Here's the drawing with two shaded views (mm, measured from the low corner). I have some questions. Coordinates: 2 decimals unless noted, no trailing zeros. Write each loop counter-clockwise with the first axis right and the second up, starting at its lowest first coordinate (ties: lowest second). Pieces come first, ordered by that corner, then holes. Notation, with made-up numbers: M -16,71.5 L 17,71.5 A31 cw 17,107.5 Z; hole C 13,-2.75 d10. An arc over 180 degrees is marked long. Answer as CSV lines item,"result". Start each with the question number.
Item 1: Suppose I cut it at B-B, the plane z = 0.4. State how many separate pieces and enclosed holes the cut face has, and give its area (3 significant figures).
Item 2: If I drill on line 1 along X through (y, z) = (82.4, 0.5); line 2 along X through (y, z) = (5, 0.9); line 3 along Y through (x, z) = (29.5, 0.45), over which ranges is the centre line in solid material (lowest first)? Write a range as [from, to].
Item 3: I'm going to push flat-ended pins straight in: P1, Ø0.8, axis at x = 40, z = 0.5, coming from the +Y side; P2, Ø0.8, axis at y = 66, z = 1, coming from the +X side; P3, Ø0.8, axis at y = 62.5, z = 1, coming from the -X side. Where does each tip first touch, or does it pass through?
Item 4: Suppose I cut it at C-C, the plane x = 12. Write out the boundary of the cut face in (y, z).
Item 5: Suppose I cut it at A-A, the plane y = 5. Write out the boundary of the cut face in (x, z).
Item 6: Suppose I cut it at D-D, the plane y = 48.5. Write out the boundary of the cut face in (x, z).
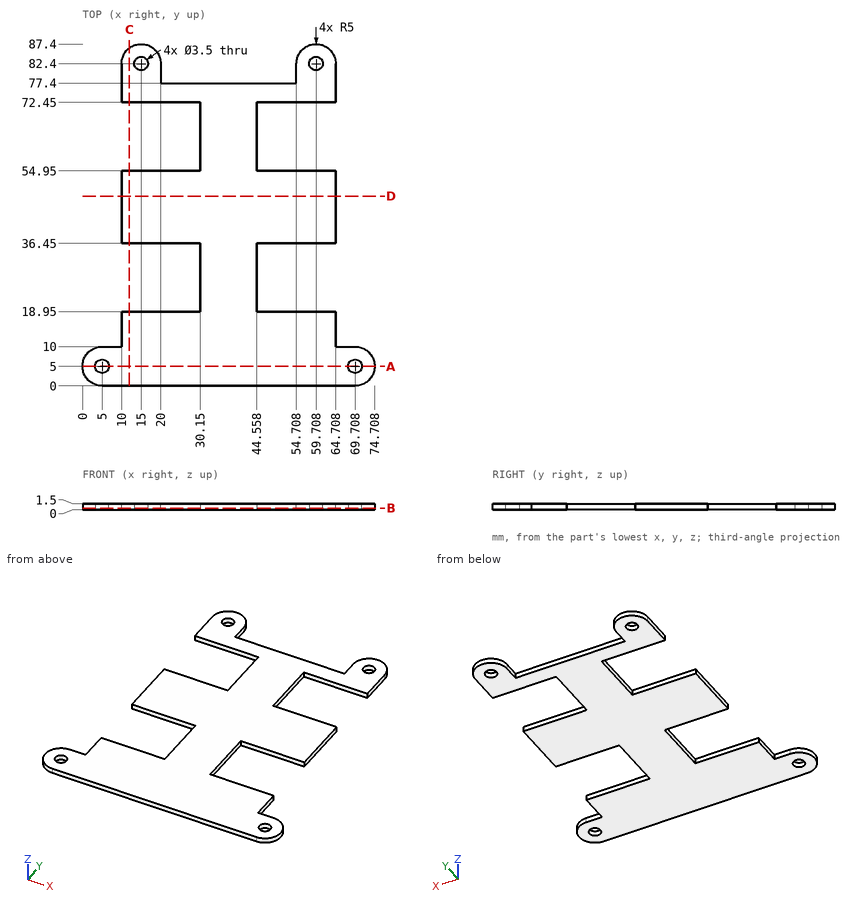
Ans:
1,separate pieces,"1"
1,enclosed holes,"4"
1,area,"3,140 mm^2"
2,line 1,"x = [10, 13.25], [16.75, 20], [54.71, 57.96], [61.46, 64.71]"
2,line 2,"x = [0, 3.25], [6.75, 67.96], [71.46, 74.71]"
2,line 3,"y = [0, 18.95], [36.45, 54.95], [72.45, 77.4]"
3,P1,"stops at y = 77.4"
3,P2,"stops at x = 44.56"
3,P3,"stops at x = 30.15"
4,outline,"M 0,0 L 18.95,0 L 18.95,1.5 L 0,1.5 Z; M 36.45,0 L 54.95,0 L 54.95,1.5 L 36.45,1.5 Z; M 72.45,0 L 86.4,0 L 86.4,1.5 L 72.45,1.5 Z"
5,outline,"M 0,0 L 3.25,0 L 3.25,1.5 L 0,1.5 Z; M 6.75,0 L 67.96,0 L 67.96,1.5 L 6.75,1.5 Z; M 71.46,0 L 74.71,0 L 74.71,1.5 L 71.46,1.5 Z"
6,outline,"M 10,0 L 64.71,0 L 64.71,1.5 L 10,1.5 Z"
